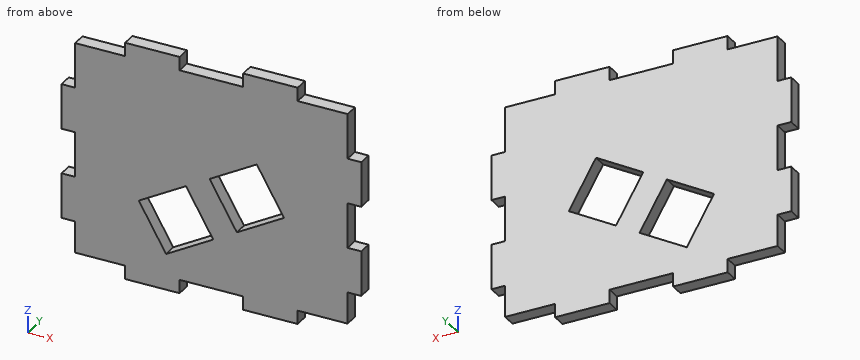
```python
from build123d import *

# Parameters (mm, degrees)
F1_DEPTH = 3


# Not quite as in the source:
# - a feature names something its author has since deleted; it is built from what else it names


with BuildPart() as f1:
    # F0 (on Front) → F1 (new body)
    with BuildSketch(Plane.XZ):
        Polygon((-19, 26.5), (-19, 23.5), (-30, 23.5), (-30, 13.5), (-33, 13.5), (-33, 3.5), (-30, 3.5), (-30, -6.5), (-33, -6.5), (-33, -16.5), (-30, -16.5), (-30, -23.5), (-19, -23.5), (-19, -26.5), (-7, -26.5), (-7, -23.5), (7, -23.5), (7, -26.5), (19, -26.5), (19, -23.5), (30, -23.5), (30, -16.5), (33, -16.5), (33, -6.5), (30, -6.5), (30, 3.5), (33, 3.5), (33, 13.5), (30, 13.5), (30, 23.5), (19, 23.5), (19, 26.5), (7, 26.5), (7, 23.5), (-7, 23.5), (-7, 26.5), align=None)
        Polygon((0.4019237886, -12.5), (-9.9903810568, -18.5), (-15.9903810568, -8.1076951546), (-5.5980762114, -2.1076951546), align=None, mode=Mode.SUBTRACT)
        Polygon((-0.4019237886, 0.8923048454), (9.9903810568, 6.8923048454), (15.9903810568, -3.5), (5.5980762114, -9.5), align=None, mode=Mode.SUBTRACT)
    extrude(amount=F1_DEPTH)


solid = f1.part
```
Verification items for the finished model (mm, model axes). Round coordinates to 2 decimals unless told otherwise and drop trailing zeros. Loops run counter-clockwise (first coordinate to the right, second up) from the corner with the lowest first, then second, coordinate; pieces in that order, holes last. Notation, with made-up numbers: (0, 74.5) -> (23, 74.5) arc R36 ccw to (23, 112.5) -> close; hole circle Ø6 at (55, 85). An arc over 180 degrees is marked (long way). Answer as a JSON object with one key per item and string values.
Q1. Go/stop test with flat-tipped pins: P1, Ø0.9, axis at y = -2, z = -1, coming from the +X side; P2, Ø0.9, axis at x = 31, y = -1.5, coming from the -Z side; P3, Ø1.5, axis at y = -1.5, z = -25, coming from the -X side; P4, Ø4, axis at x = -18.5, z = 0.5, coming from the +Y side. Record where each tip stops, or that it passes through.
Data:
{"P1": "stops at x = 30", "P2": "stops at z = -16.5", "P3": "stops at x = -19", "P4": "stops at y = 0"}
Q2. Section check A-A (y = -2.4). State how many separate pieces and enclosed holes the cut face has, then the cut area to 3 significant figures.
Data:
{"separate pieces": "1", "enclosed holes": "2", "area": "2,800 mm2"}
Q3. Scan lines: line 1 (X direction, y = -0.15, z = -24); line 2 (X direction, y = -2.1, z = -9); line 3 (Z direction, x = 27, y = -2.05). Record each from-to range of solid material in increasing order. Write a range as from..to.
Data:
{"line 1": "x = -19..-7, 7..19", "line 2": "x = -33..-15.48, -1.62..5.31, 6.46..33", "line 3": "z = -23.5..23.5"}
Q4. Section check D-D (x = 29). Record the boundary of the cut face in (y, z), then the cut area to 3 significant figures.
Data:
{"outline": "(-3, -23.5) -> (0, -23.5) -> (0, 23.5) -> (-3, 23.5) -> close", "area": "141 mm2"}
Q5. Section check B-B (x = 8). Record the boundary of the cut face in (y, z), then the cut area to 3 significant figures.
Data:
{"outline": "(-3, -26.5) -> (0, -26.5) -> (0, -8.11) -> (-3, -8.11) -> close; (-3, 5.74) -> (0, 5.74) -> (0, 26.5) -> (-3, 26.5) -> close", "area": "117 mm2"}
Q6. Section check C-C (z = 21.5). Record the boundary of the cut face in (x, y), then the cut area to 3 significant figures.
Data:
{"outline": "(-30, -3) -> (30, -3) -> (30, 0) -> (-30, 0) -> close", "area": "180 mm2"}
